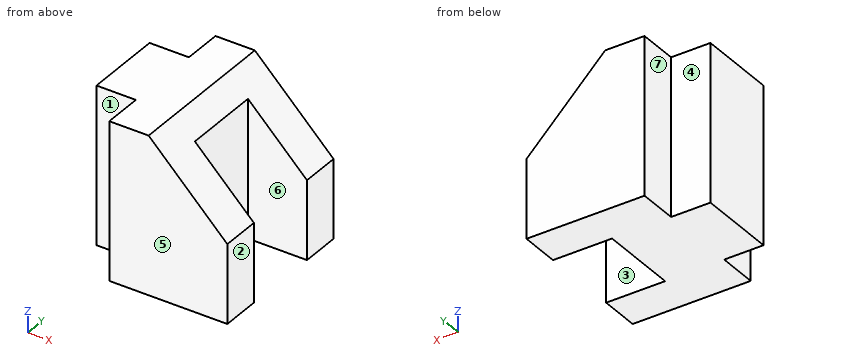
from build123d import *

# Parameters (mm, degrees)
F1_DEPTH = 25.4
F3_DEPTH = 50.801


with BuildPart() as f1:
    # F0 (on Top) → F1 (new body, symmetric)
    with BuildSketch(Plane.XY):
        Polygon((25.4, 50.8), (25.4, 0), (50.8, 0), (50.8, 12.7), (31.75, 12.7), (31.75, 38.1), (50.8, 38.1), (50.8, 50.8), align=None)
        Polygon((12.7, 12.7), (12.7, 0), (25.4, 0), (25.4, 50.8), (12.7, 50.8), (12.7, 38.1), (0, 38.1), (0, 12.7), align=None)
    extrude(amount=F1_DEPTH, both=True)

    # F2 (on face) → F3 (cut, through all)
    with BuildSketch(Plane.XZ):
        Polygon((25.4, 25.4), (50.8, 0), (50.8, 25.4), align=None)
    extrude(amount=-F3_DEPTH, mode=Mode.SUBTRACT)


solid = f1.part
For this review, take the finished solid that the model builds, in its own axes (mm). Face numbers are marked on the shaded views. A direction names the side the tool comes from. Round coordinates to 2 decimals unless told otherwise and drop trailing zeros. Order: outer loops, then holes, each group sorted by start corner. A loop starts at its lowest first (then second) coordinate and runs counter-clockwise, first axis right, second up. Notation, with made-up numbers: (69, 82) -> (116, 82) arc R23 cw to (116, 97) -> close; hole circle Ø5 at (-13.5, 19.25). An arc over 180 degrees is marked (long way). Write item = value, one per line. Start each with the question number.
1) To check wall thickness, follow line 1 (Y direction, x = 46.5, z = -12); line 2 (Y direction, x = 6, z = 1); line 3 (X direction, y = 47, z = -11). State the ranges of each line that lie inside material, in increasing order. Write a range as from..to.
2) Take a section at A-A on x = 41.5. State the section outline as (y, z) points, plus the area to 3 significant figures.
3) Take a section at B-B on z = 2.5. State the section outline as (x, y) points, plus the area to 3 significant figures.
4) The part is to be moulded in two halves that separate along Y. For the marked faces 4, 5, 6 and 7, say which applies: +Y half, -Y half, draft (parallel to the pull), parting line (faces both ways), or undercut.
5) Tool access review of the marked faces 1, 2 and 3: name each direction out of +Z, -Z, +X, -X, +Y, -Y from which nothing blocks a thin tool from reaching the whole face with its end or side.
6) Take a section at C-C on y = 24. State the section outline as (x, z) points, plus the area to 3 significant figures.
7) Insertion check: pin 1 (1 mm diameter, centred on y = 41.5, z = 17.5, fed in from +X); pin 2 (6.5 mm diameter, centred on y = 41.5, z = 1, fed in from -X); pin 3 (14 mm diameter, centred on x = 5, z = -12.5, fed in from +Y). Each pin has a flat end and moves straight along its axis. Give the tip position at first contact, or say it passes through.
8) Take a section at D-D on x = 8. State the section outline as (y, z) points.
Verdict:
q1.line_1 = 0..12.7, 38.1..50.8
q1.line_2 = 12.7..38.1
q1.line_3 = 12.7..50.8
q2.outline = (0, -25.4) -> (12.7, -25.4) -> (12.7, 9.3) -> (0, 9.3) -> close; (38.1, -25.4) -> (50.8, -25.4) -> (50.8, 9.3) -> (38.1, 9.3) -> close
q2.area = 881 mm2
q3.outline = (0, 12.7) -> (12.7, 12.7) -> (12.7, 0) -> (48.3, 0) -> (48.3, 12.7) -> (31.75, 12.7) -> (31.75, 38.1) -> (48.3, 38.1) -> (48.3, 50.8) -> (12.7, 50.8) -> (12.7, 38.1) -> (0, 38.1) -> close
q3.area = 1,710 mm2
q4.face_4 = +Y half
q4.face_5 = -Y half
q4.face_6 = undercut
q4.face_7 = draft
q5.face_1 = +Z, -Z, -X, -Y
q5.face_2 = +Z, -Z, +X, +Y, -Y
q5.face_3 = +Z, -Z, +X
q6.outline = (0, -25.4) -> (31.75, -25.4) -> (31.75, 19.05) -> (25.4, 25.4) -> (0, 25.4) -> close
q6.area = 1,590 mm2
q7.pin_1 = 33.8
q7.pin_2 = 12.7
q7.pin_3 = 38.1
q8.outline = (12.7, -25.4) -> (38.1, -25.4) -> (38.1, 25.4) -> (12.7, 25.4) -> close
